Source: CAD feature listing. Evaluate the final solid. Frame: model axes, mm. Face numbers are marked on the shaded views. Round coordinates to 2 decimals unless told otherwise and drop trailing zeros. Loops run counter-clockwise (first coordinate to the right, second up) from the corner with the lowest first, then second, coordinate; pieces in that order, holes last.
(1) First-contact query: pin 1 Ø22 at (y, z) = (-24.5, -38) entering from +X; pin 2 Ø4.5 at (x, z) = (-382, 54) entering from -Y; pin 3 Ø10 at (x, y) = (-3.5, -24) entering from +Z. Flat tips, straight axial feed; report the tip coordinate or a pass-through.
(2) Section B-B, the plane y = 15. Return the cut outline in (x, z).
(3) Section A-A, the plane z = 136. Return the cut outline in (x, y), plus the area to 3 significant figures.
(4) Mould query, pull axis X, two halves, no side actions, for the marked faces 1 and 2. Classes: pulls with the +X half, pulls with the -X half, needs draft (parallel to the pull), parting line crosses it, or undercut.
(5) Material intervals for probe 1 along X at (y, z) = (-15.5, -32); probe 2 along X at (y, z) = (-13, 60.5); probe 3 along Y at (x, z) = (48, -82.5), sorted ascending.
(6) Section C-C, the plane x = 52. Return the cut outline in (y, z), plus the area to 3 significant figures.
```python
from build123d import *

# Parameters (mm, degrees)
SKETCH1_W           = 612
SKETCH1_H           = 580
BOSS_EXTRUDE1_DEPTH = 35
FILLET9_R           = 1
CHAMFER1_SIZE       = 30
FILLET10_R          = 25
SKETCH3_W           = 37.926087763
SKETCH3_H           = 455
BOSS_EXTRUDE2_DEPTH = 35
CHAMFER2_SIZE       = 50
SKETCH4_W           = 12.193127302
SKETCH4_H           = 355
CUT_EXTRUDE1_DEPTH  = 20


with BuildPart() as part:
    # Sketch1 → Boss-Extrude1 (new body)
    with BuildSketch(Plane(origin=(0, 0, 0), x_dir=(1, 0, 0), z_dir=(0, 1, 0))):
        with Locations((-191.292576419, -30)):
            Rectangle(SKETCH1_W, SKETCH1_H)
    extrude(amount=BOSS_EXTRUDE1_DEPTH)

    # Fillet9
    fillet9_edges = [part.edges().sort_by_distance(p)[0] for p in [
        (114.707423581, 35, 30),
        (-191.292576419, 35, -260),
        (-497.292576419, 35, 30),
        (-191.292576419, 35, 320),
    ]]
    fillet(fillet9_edges, radius=FILLET9_R)

    # Chamfer1
    chamfer1_edges = [part.edges().sort_by_distance(p)[0] for p in [
        (-191.292576419, 0, 320),
    ]]
    chamfer(chamfer1_edges, length=CHAMFER1_SIZE)

    # Fillet10
    # the kernel refuses this fillet: 25 mm, written as the material it takes off along each edge
    with BuildSketch(Plane(origin=(89.707423581, 35, -235), x_dir=(1, 0, 0), z_dir=(0, 0, 1))) as fillet10_piece_1:
        with BuildLine():
            CenterArc((24, -1), 1, 0, 90)
            Line((25, -1), (25, 0))
            Line((25, 0), (24, 0))
        make_face()
    revolve(axis=Axis((89.707423581, 35, -235), (0, 1, 0)), revolution_arc=90, mode=Mode.SUBTRACT)
    with BuildSketch(Plane(origin=(-472.292576419, 35, -235), x_dir=(0, 0, -1), z_dir=(1, 0, 0))) as fillet10_piece_2:
        with BuildLine():
            CenterArc((24, -1), 1, 0, 90)
            Line((25, -1), (25, 0))
            Line((25, 0), (24, 0))
        make_face()
    revolve(axis=Axis((-472.292576419, 35, -235), (0, 1, 0)), revolution_arc=90, mode=Mode.SUBTRACT)
    with BuildSketch(Plane(origin=(-497.292576419, -62.5, -260), x_dir=(0, 0, 1), z_dir=(0, 1, 0))) as fillet10_piece_3:
        with BuildLine():
            CenterArc((FILLET10_R, FILLET10_R), FILLET10_R, 180, 90)
            Line((0, FILLET10_R), (0, 0))
            Line((0, 0), (FILLET10_R, 0))
        make_face()
    extrude(amount=97.5, mode=Mode.SUBTRACT)
    with BuildSketch(Plane(origin=(114.707423581, -62.5, -260), x_dir=(0, 0, 1), z_dir=(0, 1, 0))) as fillet10_piece_4:
        with BuildLine():
            CenterArc((FILLET10_R, -FILLET10_R), FILLET10_R, 90, 90)
            Line((0, -FILLET10_R), (0, 0))
            Line((0, 0), (FILLET10_R, 0))
        make_face()
    extrude(amount=97.5, mode=Mode.SUBTRACT)

    # Sketch3 → Boss-Extrude2 (add)
    with BuildSketch(Plane.XZ):
        with Locations((0.812875154, 2.003525588)):
            Rectangle(SKETCH3_W, SKETCH3_H)
        Polygon((-362.292576419, -224.84785724), (-402.292576419, -225.603407802), (-402.292576419, 229.396592198), (-362.292576419, 229.396592198), align=None)
    extrude(amount=BOSS_EXTRUDE2_DEPTH)

    # Chamfer2
    # the kernel refuses this chamfer: 50 mm, written as the material it takes off along each edge
    with BuildSketch(Plane(origin=(148.360068433, -35, -225.496474412), x_dir=(0, 0.9996219169112966, -0.027495876610586594), z_dir=(-1, 0, 0))) as chamfer2_piece_1_section:
        Polygon((CHAMFER2_SIZE * 0.999621916911, -CHAMFER2_SIZE * 0.0274958766106), (-CHAMFER2_SIZE * 0.0274958766106, -CHAMFER2_SIZE * 0.999621916911), (0, 0), align=None)
    chamfer2_piece_1 = extrude(amount=295.09438656, mode=Mode.PRIVATE)
    chamfer2_piece_1 = split(chamfer2_piece_1, bisect_by=Plane(origin=(0.812875153, 0, -207.548086942), z_dir=(0, -1, 0)), keep=Keep.TOP, mode=Mode.PRIVATE)
    add(chamfer2_piece_1, mode=Mode.SUBTRACT)
    with BuildSketch(Plane(origin=(-233.731359359, -35, -222.419494743), x_dir=(0.0005192705001048889, 0.9996219169112966, -0.027490972858964104), z_dir=(-0.999821655017895, 0, -0.018885395343422682))) as chamfer2_piece_2_section:
        Polygon((CHAMFER2_SIZE * 0.999621916911, -CHAMFER2_SIZE * 0.0274958766106), (-CHAMFER2_SIZE * 0.0274958766106, -CHAMFER2_SIZE * 0.999621916911), (0, 0), align=None)
    chamfer2_piece_2 = extrude(amount=297.175433868, mode=Mode.PRIVATE)
    chamfer2_piece_2 = split(chamfer2_piece_2, bisect_by=Plane(origin=(-382.631538812, 0, -207.280446055), z_dir=(0, -1, 0)), keep=Keep.TOP, mode=Mode.PRIVATE)
    add(chamfer2_piece_2, mode=Mode.SUBTRACT)
    with BuildSketch(Plane(origin=(-530.876725818, -35, 229.396592198), x_dir=(0, 0.9996219169112966, 0.027495876610586594), z_dir=(1, 0, 0))) as chamfer2_piece_3_section:
        Polygon((CHAMFER2_SIZE * 0.999621916911, -CHAMFER2_SIZE * 0.0274958766106), (-CHAMFER2_SIZE * 0.0274958766106, -CHAMFER2_SIZE * 0.999621916911), (0, 0), align=None)
    chamfer2_piece_3 = extrude(amount=297.168298797, mode=Mode.PRIVATE)
    chamfer2_piece_3 = split(chamfer2_piece_3, bisect_by=Plane(origin=(-382.292576419, 0, 211.448204728), z_dir=(0, -1, 0)), keep=Keep.TOP, mode=Mode.PRIVATE)
    add(chamfer2_piece_3, mode=Mode.SUBTRACT)
    with BuildSketch(Plane(origin=(-146.734318126, -35, 229.503525588), x_dir=(0, 0.9996219169112966, 0.027495876610586594), z_dir=(1, 0, 0))) as chamfer2_piece_4_section:
        Polygon((CHAMFER2_SIZE * 0.999621916911, -CHAMFER2_SIZE * 0.0274958766106), (-CHAMFER2_SIZE * 0.0274958766106, -CHAMFER2_SIZE * 0.999621916911), (0, 0), align=None)
    chamfer2_piece_4 = extrude(amount=295.09438656, mode=Mode.PRIVATE)
    chamfer2_piece_4 = split(chamfer2_piece_4, bisect_by=Plane(origin=(0.812875153, 0, 211.555138118), z_dir=(0, -1, 0)), keep=Keep.TOP, mode=Mode.PRIVATE)
    add(chamfer2_piece_4, mode=Mode.SUBTRACT)

    # Sketch4 → Cut-Extrude1 (cut)
    with BuildSketch(Plane.XZ.offset(35)):
        with Locations((-0.673352928, 2.003525588)):
            Rectangle(SKETCH4_W, SKETCH4_H)
        Polygon((-390.446989022, 179.396592198), (-390.446989022, -175.370740457), (-375.815236259, -175.094364731), (-375.815236259, 179.396592198), align=None)
    extrude(amount=-CUT_EXTRUDE1_DEPTH, mode=Mode.SUBTRACT)


solid = part.part
```
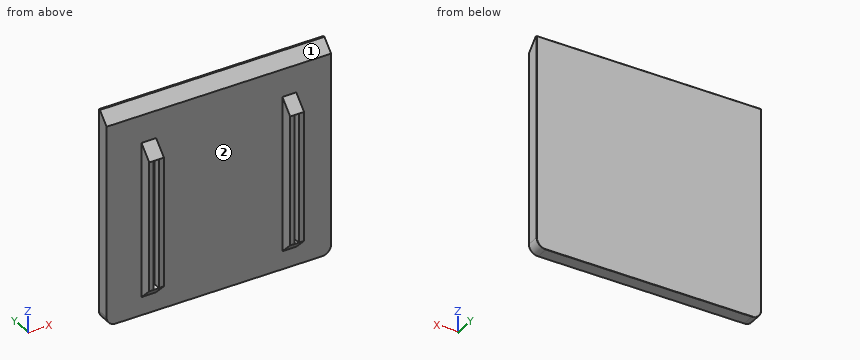
Output values:
1. pin 1: stops at x = 19.78
1. pin 2: stops at y = -15
1. pin 3: stops at z = 195.5
2. outline: (-497.29, -235) arc R25 ccw to (-472.29, -260) - (89.71, -260) arc R25 ccw to (114.71, -235) - (114.71, 305) - (-497.29, 305) - close
3. outline: (-497.29, 0) - (-402.29, 0) - (-402.29, -35) - (-390.45, -35) - (-390.45, -15) - (-375.82, -15) - (-375.82, -35) - (-362.29, -35) - (-362.29, 0) - (-18.15, 0) - (-18.15, -35) - (-6.77, -35) - (-6.77, -15) - (5.42, -15) - (5.42, -35) - (19.78, -35) - (19.78, 0) - (114.71, 0) - (114.71, 34) arc R1 ccw to (113.71, 35) - (-496.29, 35) arc R1 ccw to (-497.29, 34) - close
3. area: 23,600 mm2
4. face 1: needs draft
4. face 2: undercut
5. probe 1: x = -402.29 to -390.45, -375.82 to -362.29, -18.15 to -6.77, 5.42 to 19.78
5. probe 2: x = -402.29 to -362.29, -18.15 to 19.78
5. probe 3: y = 0 to 35
6. outline: (0, -260) - (34, -260) arc R1 ccw to (35, -259) - (35, 319) arc R1 ccw to (34, 320) - (30, 320) - (0, 290) - close
6. area: 19,800 mm2
